Drawing for the job (mm, zero at the part's lowest x, y, z). Give positions to 0.01 mm unless a question says otherwise; leave off trailing zeros. Write each loop counter-clockwise with the first axis right and the second up, starting at its lowest first coordinate (ties: lowest second). Pieces come first, ordered by that corner, then holes. Notation, with made-up numbers: (60, -34.75) - (117, -34.75) arc R9 cw to (117, -19.75) - close; hole circle Ø3 at (45, 10). An arc over 180 degrees is marked (long way). Answer as a JSON object with one key per item and string values. Group by question number.
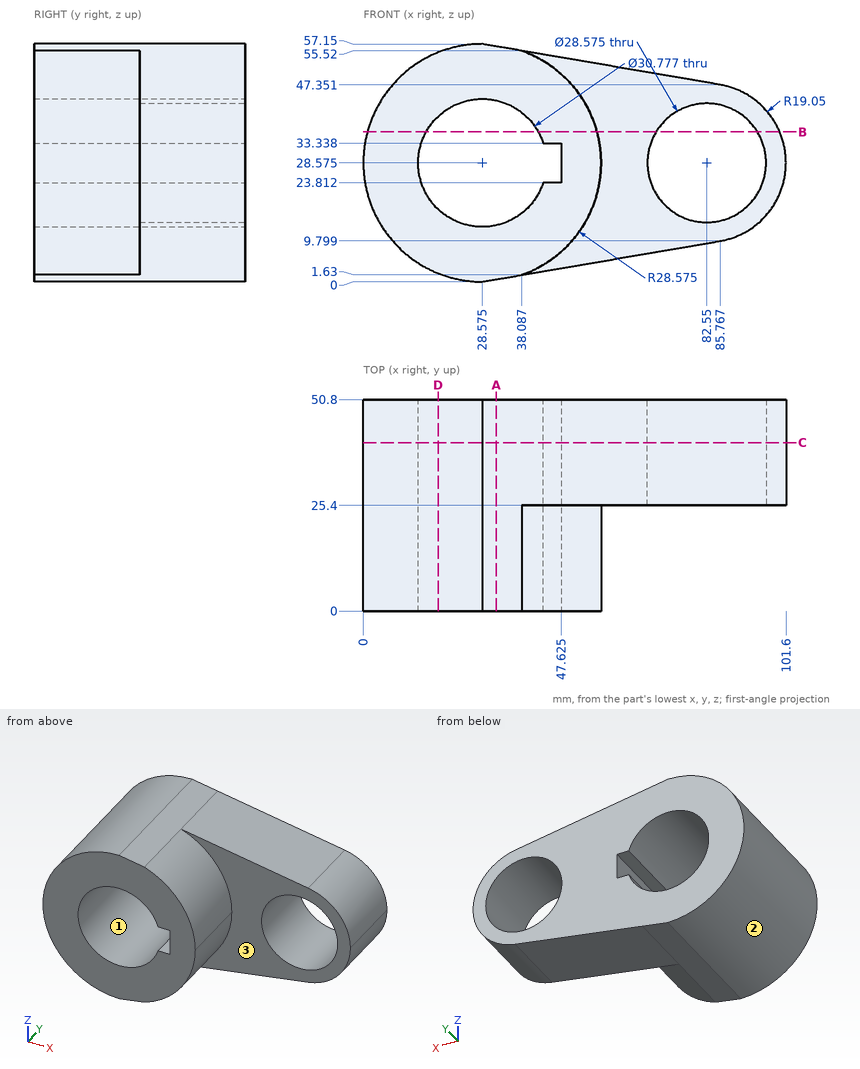
1) Band-saw the part on A-A (x = 32). List the corners of the cut face in (y, z).
2) Band-saw the part on C-C (y = 40.5). State how many separate pieces and enclosed holes the cut face has, plus the area to 3 significant figures.
3) Band-saw the part on B-B (z = 36). List the corners of the cut face in (x, y), plus the area to 3 significant figures.
4) Band-saw the part on D-D (x = 18). List the corners of the cut face in (y, z) (1 decimal), plus the area to 3 significant figures.
5) Probe line 1 (Z direction, x = 88, y = 37); line 2 (Z direction, x = 35, y = 38); line 3 (Y direction, x = 50.5, z = 6). List the from-to ranges inside material, lowest first.
6) Mould opens along X. For the marked faces 1, 2 and 3 say: pulls with the +X half, pulls with the -X half, needs draft (parallel to the pull), parting line crosses it, or undercut.
7) Drop flat-ended pins along their axis: P1, Ø24.5, axis at x = 28.575, z = 28.575, coming from the +Y side; P2, Ø6, axis at x = 18, y = 34, coming from the -Z side; P3, Ø10, axis at y = 35.5, z = 23, coming from the +X side; P4, Ø4, axis at y = 27, z = 33, coming from the +X side (1 decimal). Give the stop position or say it passes through.
Verdict:
{
 "1": {"outline": "(0, 0.59) - (50.8, 0.59) - (50.8, 13.57) - (0, 13.57) - close; (0, 43.58) - (50.8, 43.58) - (50.8, 56.56) - (0, 56.56) - close"},
 "2": {"separate pieces": "1", "enclosed holes": "2", "area": "3,020 mm2"},
 "3": {"outline": "(0.98, 0) - (15.1, 0) - (15.1, 50.8) - (0.98, 50.8) - close; (42.05, 0) - (56.17, 0) - (56.17, 25.4) - (70.34, 25.4) - (70.34, 50.8) - (42.05, 50.8) - close; (94.76, 25.4) - (100.09, 25.4) - (100.09, 50.8) - (94.76, 50.8) - close", "area": "1,930 mm2"},
 "4": {"outline": "(0, 2) - (50.8, 2) - (50.8, 17.4) - (0, 17.4) - close; (0, 39.8) - (50.8, 39.8) - (50.8, 55.1) - (0, 55.1) - close", "area": "1,560 mm2"},
 "5": {"line 1": "10.32 to 15.37, 41.78 to 46.83", "line 2": "1.1 to 14.59, 42.56 to 56.05", "line 3": "25.4 to 50.8"},
 "6": {"face 1": "undercut", "face 2": "pulls with the -X half", "face 3": "needs draft"},
 "7": {"P1": "through", "P2": "z = 1.02", "P3": "x = 101.59", "P4": "x = 101.4"}
}
